```python
from build123d import *

# Parameters (mm, degrees)
F0_W     = 2438.4
F0_H     = 1346.2
F1_DEPTH = 50.8
F2_W     = 546.1
F2_H     = 355.6
F2_H_2   = 431.8
F3_DEPTH = 177.8


with BuildPart() as f1:
    # F0 (on Top) → F1 (new body)
    with BuildSketch(Plane.XY):
        with Locations((0, 673.1)):
            Rectangle(F0_W, F0_H)
    extrude(amount=F1_DEPTH)

    # F2 (on face) → F3 (join)
    with BuildSketch(Plane.XY.offset(50.8)):
        Polygon((-1219.2, 457.2), (-1219.2, 406.4), (-1219.2, 50.8), (-1219.2, 0), (-1168.4, 0), (-622.3, 0), (-571.5, 0), (-25.4, 0), (25.4, 0), (571.5, 0), (622.3, 0), (1168.4, 0), (1219.2, 0), (1219.2, 50.8), (1219.2, 406.4), (1219.2, 457.2), (1219.2, 889), (1219.2, 939.8), (1219.2, 1295.4), (1219.2, 1346.2), (1168.4, 1346.2), (622.3, 1346.2), (571.5, 1346.2), (25.4, 1346.2), (-25.4, 1346.2), (-571.5, 1346.2), (-622.3, 1346.2), (-1168.4, 1346.2), (-1219.2, 1346.2), (-1219.2, 1295.4), (-1219.2, 939.8), (-1219.2, 889), align=None)
        with Locations((-895.35, 228.6)):
            Rectangle(F2_W, F2_H, mode=Mode.SUBTRACT)
        with Locations((-298.45, 228.6)):
            Rectangle(F2_W, F2_H, mode=Mode.SUBTRACT)
        with Locations((298.45, 228.6)):
            Rectangle(F2_W, F2_H, mode=Mode.SUBTRACT)
        with Locations((895.35, 228.6)):
            Rectangle(F2_W, F2_H, mode=Mode.SUBTRACT)
        with Locations((-895.35, 673.1)):
            Rectangle(F2_W, F2_H_2, mode=Mode.SUBTRACT)
        with Locations((-298.45, 673.1)):
            Rectangle(F2_W, F2_H_2, mode=Mode.SUBTRACT)
        with Locations((-895.35, 1117.6)):
            Rectangle(F2_W, F2_H, mode=Mode.SUBTRACT)
        with Locations((-298.45, 1117.6)):
            Rectangle(F2_W, F2_H, mode=Mode.SUBTRACT)
        with Locations((298.45, 673.1)):
            Rectangle(F2_W, F2_H_2, mode=Mode.SUBTRACT)
        with Locations((895.35, 673.1)):
            Rectangle(F2_W, F2_H_2, mode=Mode.SUBTRACT)
        with Locations((298.45, 1117.6)):
            Rectangle(F2_W, F2_H, mode=Mode.SUBTRACT)
        with Locations((895.35, 1117.6)):
            Rectangle(F2_W, F2_H, mode=Mode.SUBTRACT)
    extrude(amount=F3_DEPTH)


solid = f1.part
```
Geometry check sheet. Reference: the model listing, model coordinates, mm. Round coordinates to 2 decimals unless told otherwise and drop trailing zeros. Order: outer loops, then holes, each group sorted by start corner. A loop starts at its lowest first (then second) coordinate and runs counter-clockwise, first axis right, second up. Notation, with made-up numbers: M -31.5,-0.5 L -19.5,-0.5 A29 ccw -19.5,21.5 Z; hole C 22.5,27 d2. An arc over 180 degrees is marked long. Write item = value, one per line.
Q1. Depth check by flat-ended pin: pin 1 Ø1 at (x, y) = (518.5, 750) entering from +Z. Enter the tip coordinate at first touch or a pass-through.
Answer block:
pin_1 = 50.8
Q2. Scan lines: line 1 (Y direction, x = 464, z = 124); line 2 (X direction, y = 621, z = 158); line 3 (Z direction, x = 1038.5, y = 305). Record each from-to range of solid material in increasing order.
Answer block:
line_1 = 0 to 50.8, 406.4 to 457.2, 889 to 939.8, 1295.4 to 1346.2
line_2 = -1219.2 to -1168.4, -622.3 to -571.5, -25.4 to 25.4, 571.5 to 622.3, 1168.4 to 1219.2
line_3 = 0 to 50.8
Q3. Release check for a two-part mould opening along Y. For faces 1 (the flat face through (-17, 0, 113)), 2 (the flat face through (1168.4, 1115, 138)) record: released by +Y, released by -Y, zero draft, split by the parting line, or undercut.
Answer block:
face_1 = released by -Y
face_2 = undercut
Q4. Section check C-C (z = 197.5). Give the number of separate pieces and of enclosed holes in the cut face, plus the area to 3 significant figures.
Answer block:
separate_pieces = 1
enclosed_holes = 12
area = 786,000 mm^2
Q5. Section check A-A (x = 258). Enter the section's corners in (y, z).
Answer block:
outline = M 0,0 L 1346.2,0 L 1346.2,228.6 L 1295.4,228.6 L 1295.4,50.8 L 939.8,50.8 L 939.8,228.6 L 889,228.6 L 889,50.8 L 457.2,50.8 L 457.2,228.6 L 406.4,228.6 L 406.4,50.8 L 50.8,50.8 L 50.8,228.6 L 0,228.6 Z
Q6. Section check B-B (y = 633). Enter the section's corners in (x, z).
Answer block:
outline = M -1219.2,0 L 1219.2,0 L 1219.2,228.6 L 1168.4,228.6 L 1168.4,50.8 L 622.3,50.8 L 622.3,228.6 L 571.5,228.6 L 571.5,50.8 L 25.4,50.8 L 25.4,228.6 L -25.4,228.6 L -25.4,50.8 L -571.5,50.8 L -571.5,228.6 L -622.3,228.6 L -622.3,50.8 L -1168.4,50.8 L -1168.4,228.6 L -1219.2,228.6 Z
